CAD build for the part. Positions are in the model's coordinates, mm. A direction names the side the tool comes from. Coordinates: 2 decimals unless noted, no trailing zeros. Loops run counter-clockwise (first coordinate to the right, second up) from the corner with the lowest first, then second, coordinate; pieces in that order, holes last. Notation, with made-up numbers: (-34, 82) - (-17, 82) arc R15 cw to (-17, 99) - close; hole circle Ø5 at (67, -29). An arc over 180 degrees is marked (long way). Put each result on its own line as item: value.
```python
from build123d import *

# Parameters (mm, degrees)
SKETCH3_W           = 18
SKETCH3_H           = 20
SKETCH3_R           = 2.125
BOSS_EXTRUDE3_DEPTH = 2.75
SKETCH5_W           = 20
SKETCH5_H           = 15
SKETCH5_R           = 2.125
BOSS_EXTRUDE5_DEPTH = 2.75
FILLET4_R           = 2


with BuildPart() as part:
    # Sketch3 → Boss-Extrude3 (new body)
    with BuildSketch(Plane(origin=(0, 0, 0), x_dir=(1, 0, 0), z_dir=(0, 1, 0))):
        with Locations((6, 0)):
            Rectangle(SKETCH3_W, SKETCH3_H)
        with Locations(Location((10, 6, 0), (0, 0, 270))):
            Circle(SKETCH3_R, mode=Mode.SUBTRACT)
        with Locations(Location((10, -6, 0), (0, 0, 90))):
            Circle(SKETCH3_R, mode=Mode.SUBTRACT)
    extrude(amount=BOSS_EXTRUDE3_DEPTH)

    # Sketch5 → Boss-Extrude5 (add)
    with BuildSketch(Plane.ZY.offset(3)):
        with Locations((0, 7.5)):
            Rectangle(SKETCH5_W, SKETCH5_H)
        with Locations((-6, 10)):
            Circle(SKETCH5_R, mode=Mode.SUBTRACT)
        with Locations(Location((6, 10, 0), (0, 0, 180))):
            Circle(SKETCH5_R, mode=Mode.SUBTRACT)
    extrude(amount=-BOSS_EXTRUDE5_DEPTH)

    # Fillet4
    fillet4_edges = [part.edges().sort_by_distance(p)[0] for p in [
        (-1.625, 15, 10),
        (-1.625, 15, -10),
        (-0.25, 2.75, 0),
        (15, 1.375, 10),
        (15, 1.375, -10),
    ]]
    fillet(fillet4_edges, radius=FILLET4_R)


solid = part.part
```
Q1. Slice it at C-C, the plane x = 10. Give the cut face in (y, z) (3 decimals), then the cut area to 3 significant figures.
Determined:
outline: (0, -10) - (2.75, -10) - (2.75, -8.125) - (0, -8.125) - close; (0, -3.875) - (2.75, -3.875) - (2.75, 3.875) - (0, 3.875) - close; (0, 8.125) - (2.75, 8.125) - (2.75, 10) - (0, 10) - close
area: 31.6 mm2
Q2. Wall check: L1, parallel to Y at x = -1.1, z = 6 (3 decimals); L2, parallel to X at y = 1.9, z = -6 (3 decimals); L3, parallel to X at y = 12.5, z = 2.25. Give the ranges that are in metal, low to high. Write a range as from..to.
Determined:
L1: 0..7.875, 12.125..15
L2: -3..7.875, 12.125..15
L3: -3..-0.25
Q3. Mould opens along Z. For faces 1 (the cylindrical face through (14.43, 1.39, -9.4)), 2 (the cylindrical face through (-1.61, 14.43, 9.4)), 3 (the cylindrical face through (7.926, 1.356, -6.461)) say: +Z half, -Z half, draft (parallel to the pull), parting line (faces both ways), or undercut.
Determined:
face 1: -Z half
face 2: +Z half
face 3: undercut
Q4. Slice it at D-D, the plane y = 10. Give the cut face in (x, z) (3 decimals).
Determined:
outline: (-3, -10) - (-0.25, -10) - (-0.25, -8.125) - (-3, -8.125) - close; (-3, -3.875) - (-0.25, -3.875) - (-0.25, 3.875) - (-3, 3.875) - close; (-3, 8.125) - (-0.25, 8.125) - (-0.25, 10) - (-3, 10) - close
Q5. Pin check, flat tips, straight feed: pin 1 Ø1 at (x, z) = (-1, 0.5) entering from -Y; pin 2 Ø3.5 at (x, z) = (10, -6) entering from +Y; pin 3 Ø1 at (x, z) = (4.5, 3.5) entering from +Y; pin 4 Ø3 at (y, z) = (10.5, 5) entering from +X. Stop position of each tip, or through.
Determined:
pin 1: y = 0
pin 2: through
pin 3: y = 2.75
pin 4: x = -0.25
Q6. Tool access for faces 4 (the flat face through (-3, 7, 0)), 5 (the flat face through (8, 2.75, 0)): list every direction of +Z, -Z, +X, -X, +Y, -Y with a clear straight run to the whole face (end or side of a thin tool).
Determined:
face 4: +Z, -Z, -X, +Y, -Y
face 5: +Z, -Z, +X, +Y
Q7. Slice it at B-B, the plane y = 1.5. Give the cut face in (x, z) (3 decimals), then the cut area to 3 significant figures.
Determined:
outline: (-3, -10) - (13, -10) arc R2 ccw to (15, -8) - (15, 8) arc R2 ccw to (13, 10) - (-3, 10) - close; hole circle Ø4.25 at (10, -6); hole circle Ø4.25 at (10, 6)
area: 330 mm2
Q8. Slice it at A-A, the plane z = 6. Give the cut face in (x, y) (3 decimals).
Determined:
outline: (-3, 0) - (7.875, 0) - (7.875, 2.75) - (1.75, 2.75) arc R2 cw to (-0.25, 4.75) - (-0.25, 7.875) - (-3, 7.875) - close; (-3, 12.125) - (-0.25, 12.125) - (-0.25, 15) - (-3, 15) - close; (12.125, 0) - (15, 0) - (15, 2.75) - (12.125, 2.75) - close
